```python
from build123d import *

# Parameters (mm, degrees)
ESBO_O1_R                = 20
ESBO_O1_R_2              = 2.85
ESBO_O1_R_3              = 2
RESSALTO_EXTRUS_O1_DEPTH = 3


with BuildPart() as part:
    # Esboço1 → Ressalto-extrusão1 (new body)
    with BuildSketch(Plane.XZ.offset(3)):
        with Locations(Location((0, 0, 0), (0, 0, 90))):
            Circle(ESBO_O1_R)
        with Locations(Location((0, 0, 0), (0, 0, 90))):
            Circle(ESBO_O1_R_2, mode=Mode.SUBTRACT)
        with Locations(Location((10.557104243, 10.557104243, 0), (0, 0, 90))):
            Circle(ESBO_O1_R_3, mode=Mode.SUBTRACT)
        with Locations(Location((10.557104243, -10.557104243, 0), (0, 0, 90))):
            Circle(ESBO_O1_R_3, mode=Mode.SUBTRACT)
        with Locations(Location((-10.557104243, -10.557104243, 0), (0, 0, 90))):
            Circle(ESBO_O1_R_3, mode=Mode.SUBTRACT)
        with Locations(Location((-10.557104243, 10.557104243, 0), (0, 0, 90))):
            Circle(ESBO_O1_R_3, mode=Mode.SUBTRACT)
    extrude(amount=-RESSALTO_EXTRUS_O1_DEPTH)


solid = part.part
```
Work out the finished part from the listing and answer in its coordinate system (mm). Round coordinates to 2 decimals unless told otherwise and drop trailing zeros. Loops run counter-clockwise (first coordinate to the right, second up) from the corner with the lowest first, then second, coordinate; pieces in that order, holes last.
(1) The part is cut by section C-C, the plane z = 11.5. Give the vertices of the cut face in (x, y), and give its area (3 significant figures).
Computed values:
outline: (-16.36, -3) - (-12.32, -3) - (-12.32, 0) - (-16.36, 0) - close; (-8.79, -3) - (8.79, -3) - (8.79, 0) - (-8.79, 0) - close; (12.32, -3) - (16.36, -3) - (16.36, 0) - (12.32, 0) - close
area: 77.0 mm2
(2) The part is cut by section A-A, the plane z = 0. Give the vertices of the cut face in (x, y).
Computed values:
outline: (-20, -3) - (-2.85, -3) - (-2.85, 0) - (-20, 0) - close; (2.85, -3) - (20, -3) - (20, 0) - (2.85, 0) - close
(3) Find the intervals of material crossed by L1, parallel to X at y = -1.5, z = 11; L2, parallel to X at y = -1.5, z = 0; L3, parallel to Z at x = 2.5, y = -0.3, in increasing order.
Computed values:
L1: x = -16.7 to -12.51, -8.61 to 8.61, 12.51 to 16.7
L2: x = -20 to -2.85, 2.85 to 20
L3: z = -19.84 to -1.37, 1.37 to 19.84
(4) The part is cut by section D-D, the plane y = -0.8. Give the vertices of the cut face in (x, z).
Computed values:
outline: circle Ø40 at (0, 0); hole circle Ø4 at (-10.56, -10.56); hole circle Ø4 at (-10.56, 10.56); hole circle Ø5.7 at (0, 0); hole circle Ø4 at (10.56, -10.56); hole circle Ø4 at (10.56, 10.56)
(5) The mould has two halves that part along Z. Classify faces 1 (the cylindrical face through (19.524, -1.521, -4.336)), 2 (the cylindrical face through (-12.54, -1.52, 10.3)), 3 (the flat face through (0, 0, 4)), 4 (the cylindrical face through (12.51, -1.52, 10.12)): pulls with the +Z half, pulls with the -Z half, needs draft (parallel to the pull), parting line crosses it, or undercut.
Computed values:
face 1: parting line crosses it
face 2: undercut
face 3: needs draft
face 4: undercut
(6) The part is cut by section B-B, the plane x = 0. Give the vertices of the cut face in (y, z).
Computed values:
outline: (-3, -20) - (0, -20) - (0, -2.85) - (-3, -2.85) - close; (-3, 2.85) - (0, 2.85) - (0, 20) - (-3, 20) - close
